The listing builds one solid part. Answer for the finished solid, in the listing's coordinates (mm). A direction names the side the tool comes from. Round coordinates to 2 decimals unless told otherwise and drop trailing zeros. Write each loop counter-clockwise with the first axis right and the second up, starting at its lowest first coordinate (ties: lowest second). Pieces come first, ordered by that corner, then holes. Notation, with made-up numbers: (-1, 15.25) - (5, 15.25) arc R19 cw to (5, 52.25) - close; hole circle Ø2 at (46.25, 79.5). An arc over 180 degrees is marked (long way). Use a Markdown table: item, result. Add a question column.
1) Determine the mould class of faces 1 (the flat face through (50.7, 1.9, 3.5)), 2 (the cylindrical face through (107.13, 1.42, -74.38)), 3 (the flat face through (-58, 3.81, -2)) for opening direction Y: +Y half, -Y half, draft (parallel to the pull), parting line (faces both ways), or undercut.
2) Each of these flat-tipped pins is pushed along its axis until it touches: P1, Ø1.5, axis at y = 1, z = -37, coming from the -X side; P2, Ø1.9, axis at x = 0, y = 2, coming from the -Z side; P3, Ø2, axis at x = 11.71, y = 1.9, coming from the +Z side; P4, Ø5, axis at x = -0.03, z = 94.7, coming from the -Y side. Where does it stop, or does it pass through?
3) A cutting plane is placed at B-B (z = -32.5). Give the vertices of the cut face in (x, y).
4) A cutting plane is placed at C-C (z = -95). State how many separate pieces and enclosed holes the cut face has, then the cut area to 3 significant figures.
5) A tool of negligible diameter and unlimited length cuts with its end or side. For faces 4 (the cylindrical face through (-10.326, 1.878, 68.267)), 5 (the flat face through (81.7, 1.9, 20.7)), from which of +Z, -Z, +X, -X, +Y, -Y can it reach the whole face along a straight path? Write none if from no direction.
6) A cutting plane is placed at A-A (z = 10.5). Give the vertices of the cut face in (x, y), then the cut area to 3 significant figures.
7) Find the intervals of material crossed by probe 1 along X at (y, z) = (2.25, 93); probe 2 along X at (y, z) = (0.9, 96.5); probe 3 along Z at (x, y) = (-3.5, 0.65), in increasing order. Write a range as from..to.
```python
from build123d import *

# Parameters (mm, degrees)
SKETCH1_R           = 3.175
BOSS_EXTRUDE1_DEPTH = 3.81
CUT_EXTRUDE1_REACH  = 334.908
SKETCH3_R           = 1.27
CUT_EXTRUDE2_REACH  = 274.112
SKETCH5_R           = 1.27
CUT_EXTRUDE3_REACH  = 334.911
SKETCH6_R           = 1.27


with BuildPart() as part:
    # Sketch1 → Boss-Extrude1 (new body)
    with BuildSketch(Plane(origin=(0, 0, 0), x_dir=(1, 0, 0), z_dir=(0, 1, 0))):
        with BuildLine():
            Line((-132.862230357, 80.626602679), (-114.818360917, 111.876376892))
            ThreePointArc((-114.818360917, 111.876376892), (-110.170255519, 116.524341207), (-103.82099168, 118.225900714))
            Line((-103.82099168, 118.225900714), (103.762977343, 118.240259528))
            ThreePointArc((103.762977343, 118.240259528), (110.109496385, 116.541297953), (114.757781541, 111.898214981))
            Line((114.757781541, 111.898214981), (132.857908371, 80.600189632))
            ThreePointArc((132.857908371, 80.600189632), (134.563982049, 74.246129937), (132.86180691, 67.891024761))
            Line((132.86180691, 67.891024761), (29.0379736, -111.891469007))
            ThreePointArc((29.0379736, -111.891469007), (24.389544583, -116.539131318), (18.040149336, -118.240259558))
            Line((18.040149336, -118.240259558), (-18.094408415, -118.240259558))
            ThreePointArc((-18.094408415, -118.240259558), (-24.445497205, -116.538153501), (-29.09418809, -111.888081791))
            Line((-29.09418809, -111.888081791), (-132.863762321, 67.928304298))
            ThreePointArc((-132.863762321, 67.928304298), (-134.563982554, 74.277658701), (-132.862230357, 80.626602679))
        make_face()
        with Locations(Location((-103.330851621, 84.381028983, 0), (0, 0, 90))):
            Circle(SKETCH1_R, mode=Mode.SUBTRACT)
        with Locations(Location((-0.028433279, -94.702561062, 0), (0, 0, 90))):
            Circle(SKETCH1_R, mode=Mode.SUBTRACT)
        with Locations(Location((103.336854698, 84.397127461, 0), (0, 0, 90))):
            Circle(SKETCH1_R, mode=Mode.SUBTRACT)
        with BuildLine():
            Line((-84.013266269, 67.022348434), (-78.642736989, 76.323448067))
            ThreePointArc((-78.642736989, 76.323448067), (-73.995553024, 80.970880326), (-67.647495776, 82.672971564))
            Line((-67.647495776, 82.672971564), (67.773359352, 82.705030032))
            ThreePointArc((67.773359352, 82.705030032), (74.121084724, 81.006600385), (78.770291575, 76.36298581))
            Line((78.770291575, 76.36298581), (84.141622987, 67.075091406))
            ThreePointArc((84.141622987, 67.075091406), (85.847697169, 60.718674744), (84.143163353, 54.361844845))
            Line((84.143163353, 54.361844845), (16.352129804, -62.925309178))
            ThreePointArc((16.352129804, -62.925309178), (11.704017593, -67.570067982), (5.356663713, -69.27001804))
            Line((5.356663713, -69.27001804), (-5.379766134, -69.27001804))
            ThreePointArc((-5.379766134, -69.27001804), (-11.731679612, -67.567435699), (-16.380497701, -62.916190507))
            Line((-16.380497701, -62.916190507), (-84.015750126, 54.325699819))
            ThreePointArc((-84.015750126, 54.325699819), (-85.715018316, 60.674356799), (-84.013266269, 67.022348434))
        make_face(mode=Mode.SUBTRACT)
    extrude(amount=BOSS_EXTRUDE1_DEPTH)

    # Sketch3 → Cut-Extrude1 (cut, up to next)
    with BuildSketch(Plane(origin=(134.490180652, 0, -77.777728789), x_dir=(-0.5006264112230908, 0, -0.8656634429071663), z_dir=(0.8656634429071663, 0, -0.5006264112230908)), mode=Mode.PRIVATE) as cut_extrude1_sk1:
        with Locations((9.583713099, 1.905)):
            Circle(SKETCH3_R)
    cut_extrude1_tool1 = extrude(cut_extrude1_sk1.sketch, amount=-CUT_EXTRUDE1_REACH, mode=Mode.PRIVATE) & part.part
    # Sketch3 → Cut-Extrude1 (cut, up to next)
    with BuildSketch(Plane(origin=(134.490180652, 0, -77.777728789), x_dir=(-0.5006264112230908, 0, -0.8656634429071663), z_dir=(0.8656634429071663, 0, -0.5006264112230908)), mode=Mode.PRIVATE) as cut_extrude1_sk2:
        with Locations((33.073860572, 1.905)):
            Circle(SKETCH3_R)
    cut_extrude1_tool2 = extrude(cut_extrude1_sk2.sketch, amount=-CUT_EXTRUDE1_REACH, mode=Mode.PRIVATE) & part.part
    add(cut_extrude1_tool1.solids().sort_by_distance((129.692321, 1.905, -86.073999))[0], mode=Mode.SUBTRACT)
    add(cut_extrude1_tool2.solids().sort_by_distance((117.932533, 1.905, -106.408561))[0], mode=Mode.SUBTRACT)

    # Sketch5 → Cut-Extrude2 (cut, up to next)
    with BuildSketch(Plane.XY.offset(118.240259558), mode=Mode.PRIVATE) as cut_extrude2_sk1:
        with Locations((-11.784935705, 1.905)):
            Circle(SKETCH5_R)
    cut_extrude2_tool1 = extrude(cut_extrude2_sk1.sketch, amount=-CUT_EXTRUDE2_REACH, mode=Mode.PRIVATE) & part.part
    # Sketch5 → Cut-Extrude2 (cut, up to next)
    with BuildSketch(Plane.XY.offset(118.240259558), mode=Mode.PRIVATE) as cut_extrude2_sk2:
        with Locations((11.705218914, 1.905)):
            Circle(SKETCH5_R)
    cut_extrude2_tool2 = extrude(cut_extrude2_sk2.sketch, amount=-CUT_EXTRUDE2_REACH, mode=Mode.PRIVATE) & part.part
    add(cut_extrude2_tool1.solids().sort_by_distance((-11.784936, 1.905, 118.24026))[0], mode=Mode.SUBTRACT)
    add(cut_extrude2_tool2.solids().sort_by_distance((11.705219, 1.905, 118.24026))[0], mode=Mode.SUBTRACT)

    # Sketch6 → Cut-Extrude3 (cut, up to next)
    with BuildSketch(Plane(origin=(-134.555779523, 0, -77.693582727), x_dir=(-0.500037491916206, 0, 0.8660037567344326), z_dir=(-0.8660037567344328, 0, -0.500037491916206)), mode=Mode.PRIVATE) as cut_extrude3_sk1:
        with Locations((-33.174438242, 1.905)):
            Circle(SKETCH6_R)
    cut_extrude3_tool1 = extrude(cut_extrude3_sk1.sketch, amount=-CUT_EXTRUDE3_REACH, mode=Mode.PRIVATE) & part.part
    # Sketch6 → Cut-Extrude3 (cut, up to next)
    with BuildSketch(Plane(origin=(-134.555779523, 0, -77.693582727), x_dir=(-0.500037491916206, 0, 0.8660037567344326), z_dir=(-0.8660037567344328, 0, -0.500037491916206)), mode=Mode.PRIVATE) as cut_extrude3_sk2:
        with Locations((-9.684283586, 1.905)):
            Circle(SKETCH6_R)
    cut_extrude3_tool2 = extrude(cut_extrude3_sk2.sketch, amount=-CUT_EXTRUDE3_REACH, mode=Mode.PRIVATE) & part.part
    add(cut_extrude3_tool1.solids().sort_by_distance((-117.967317, 1.905, -106.422771))[0], mode=Mode.SUBTRACT)
    add(cut_extrude3_tool2.solids().sort_by_distance((-129.713275, 1.905, -86.080209))[0], mode=Mode.SUBTRACT)


solid = part.part
```
Entries:
| question | item | result |
|---|---|---|
| 1 | face 1 | draft |
| 1 | face 2 | undercut |
| 1 | face 3 | +Y half |
| 2 | P1 | stops at x = -115.45 |
| 2 | P2 | stops at z = -118.23 |
| 2 | P3 | stops at z = -82.69 |
| 2 | P4 | passes through |
| 3 | outline | (-112.42, 0) - (-71.42, 0) - (-71.42, 3.81) - (-112.42, 3.81) - close; (71.51, 0) - (112.42, 0) - (112.42, 3.81) - (71.51, 3.81) - close |
| 4 | separate pieces | 1 |
| 4 | enclosed holes | 2 |
| 4 | area | 929 mm² |
| 5 | face 4 | +Y, -Y |
| 5 | face 5 | +Z, +X, +Y, -Y |
| 6 | outline | (-87.6, 0) - (-46.62, 0) - (-46.62, 3.81) - (-87.6, 3.81) - close; (46.65, 0) - (87.59, 0) - (87.59, 3.81) - (46.65, 3.81) - close |
| 6 | area | 312 mm² |
| 7 | probe 1 | x = -39.99..-13.01, -10.56..-2.71, 2.65..10.48, 12.93..39.95 |
| 7 | probe 2 | x = -37.97..-12.56, -11.01..-2.65, 2.59..10.93, 12.48..37.93 |
| 7 | probe 3 | z = -118.23..-82.69, 69.27..118.24 |
